Here's how the part is built. I have some questions about the finished solid (model axes, mm). A direction names the side the tool comes from. Give positions to 0.01 mm unless a question says otherwise; leave off trailing zeros. Write each loop counter-clockwise with the first axis right and the second up, starting at its lowest first coordinate (ties: lowest second). Pieces come first, ordered by that corner, then holes. Notation, with made-up numbers: (45.25, -13) -> (87.25, -13) arc R20 ccw to (87.25, 18) -> close; hole circle Ø10 at (6, 38). An arc over 180 degrees is marked (long way). Answer as CSV lines item,"result". Start each with the question number.
from build123d import *

# Parameters (mm, degrees)
BOSS_EXTRUDE1_DEPTH = 50
FILLET2_R           = 25
FILLET3_R           = 25
FILLET4_R           = 25
FILLET5_R           = 25
SKETCH2_R           = 15.5
CUT_EXTRUDE1_DEPTH  = 191.136542592
SKETCH3_R           = 25
BOSS_EXTRUDE2_DEPTH = 5
SKETCH4_R           = 6
BOSS_EXTRUDE3_DEPTH = 40
FILLET6_R           = 2
FILLET7_R           = 5


with BuildPart() as part:
    # Sketch1 → Boss-Extrude1 (new body)
    with BuildSketch(Plane.XY):
        Polygon((15, 8.751233612), (15, 118.751233612), (105, 118.751233612), (105, 8.751233612), (120, 8.751233612), (120, 138.751233612), (0, 138.751233612), (0, 8.751233612), align=None)
    extrude(amount=BOSS_EXTRUDE1_DEPTH)

    # Fillet2
    fillet2_edges = [part.edges().sort_by_distance(p)[0] for p in [
        (7.5, 8.751233612, 50),
    ]]
    fillet(fillet2_edges, radius=FILLET2_R)

    # Fillet3
    fillet3_edges = [part.edges().sort_by_distance(p)[0] for p in [
        (7.5, 8.751233612, 0),
    ]]
    fillet(fillet3_edges, radius=FILLET3_R - 0.0001)  # a hair under: the kernel refuses the full size

    # Fillet4
    fillet4_edges = [part.edges().sort_by_distance(p)[0] for p in [
        (112.5, 8.751233612, 50),
    ]]
    fillet(fillet4_edges, radius=FILLET4_R)

    # Fillet5
    fillet5_edges = [part.edges().sort_by_distance(p)[0] for p in [
        (112.5, 8.751233612, 0),
    ]]
    fillet(fillet5_edges, radius=FILLET5_R - 0.0001)  # a hair under: the kernel refuses the full size

    # Sketch2 → Cut-Extrude1 (cut, through all)
    with BuildSketch(Plane(origin=(120, 0, 0), x_dir=(0, 0, -1), z_dir=(1, 0, 0))):
        with Locations((-25, 33.751233612)):
            Circle(SKETCH2_R)
    extrude(amount=-CUT_EXTRUDE1_DEPTH, mode=Mode.SUBTRACT)

    # Sketch3 → Boss-Extrude2 (add)
    with BuildSketch(Plane(origin=(0, 138.751233612, 0), x_dir=(1, 0, 0), z_dir=(0, 1, 0))):
        with Locations(Location((60, -25, 0), (0, 0, 270))):
            Circle(SKETCH3_R)
    extrude(amount=BOSS_EXTRUDE2_DEPTH)

    # Sketch4 → Boss-Extrude3 (add)
    with BuildSketch(Plane(origin=(0, 143.751233612, 0), x_dir=(1, 0, 0), z_dir=(0, 1, 0))):
        with Locations(Location((60, -25, 0), (0, 0, 270))):
            Circle(SKETCH4_R)
    extrude(amount=BOSS_EXTRUDE3_DEPTH)

    # Fillet6
    fillet6_edges = [part.edges().sort_by_distance(p)[0] for p in [
        (60, 143.751233612, 0),
        (60, 143.751233612, 19),
    ]]
    fillet(fillet6_edges, radius=FILLET6_R)

    # Fillet7
    fillet7_edges = [part.edges().sort_by_distance(p)[0] for p in [
        (15, 118.751233612, 25),
        (0, 138.751233612, 25),
        (120, 138.751233612, 25),
        (105, 118.751233612, 25),
    ]]
    fillet(fillet7_edges, radius=FILLET7_R)


solid = part.part
Item 1: If we section it at C-C (z = 27): State how many separate pieces and enclosed holes the cut face has, and give its area (3 significant figures).
Item 2: If we section it at B-B (y = 30): Please give me the cut outline in (x, z).
Item 3: If we section it at D-D (x = 94): Please give me the cut outline in (y, z), and give its area (3 significant figures).
Item 4: We'd pull the mould along Z, two halves only. Please class faces 1 (the face through (60, 143.751, 35)), 2 (the face through (59, 122, 50)), 3 (the face through (7.61, 49.12, 27.02)): released by +Z, released by -Z, zero draft, split by the parting line, or undercut.
Item 5: If I drill on line 1 (X direction, y = 81.5, z = 26.5); line 2 (Y direction, x = 52, z = 37); line 3 (Y direction, x = 98.5, z = 21.5), over which ranges is the centre line in solid material (lowest first)? Write a range as [from, to].
Item 6: For faces 4 (the face through (112.6, 15.9, 7.5)), 5 (the face through (15, 72, 25)), 6 (the face through (64.06, 164.49, 20.58)), which set-ups out of +Z, -Z, +X, -X, +Y, -Y let a thin tool reach every point of the face, with its end or its side?
Item 7: I'm going to push flat-ended pins straight in: pin 1 (4 mm diameter, centred on x = 78.5, z = 14.5, fed in from -Y); pin 2 (25 mm diameter, centred on y = 33.75, z = 25, fed in from -X); pin 3 (25 mm diameter, centred on x = 39, z = 29, fed in from +Y); pin 4 (3 mm diameter, centred on x = 104, z = 27.5, fed in from -Y). Where does each tip first touch, or does it pass through?
Item 8: If we section it at A-A (y = 66.5): Please give me the cut outline in (x, z).
Final values:
1,separate pieces,"3"
1,enclosed holes,"0"
1,area,"5,480 mm2"
2,outline,"(0, 0.28) -> (15, 0.28) -> (15, 9.96) -> (0, 9.96) -> close; (0, 40.04) -> (15, 40.04) -> (15, 49.72) -> (0, 49.72) -> close; (105, 0.28) -> (120, 0.28) -> (120, 9.96) -> (105, 9.96) -> close; (105, 40.04) -> (120, 40.04) -> (120, 49.72) -> (105, 49.72) -> close"
3,outline,"(118.75, 0) -> (138.75, 0) -> (138.75, 50) -> (118.75, 50) -> close"
3,area,"1,000 mm2"
4,face 1,"zero draft"
4,face 2,"released by +Z"
4,face 3,"undercut"
5,line 1,"[0, 15], [105, 120]"
5,line 2,"[118.75, 143.75]"
5,line 3,"[118.75, 138.75]"
6,face 4,"-Z, +X, -X, -Y"
6,face 5,"+Z, -Z, -Y"
6,face 6,"+Y"
7,pin 1,"y = 118.75"
7,pin 2,"through"
7,pin 3,"y = 143.75"
7,pin 4,"y = 8.79"
8,outline,"(0, 0) -> (15, 0) -> (15, 50) -> (0, 50) -> close; (105, 0) -> (120, 0) -> (120, 50) -> (105, 50) -> close"
